For this review, take the finished solid that the model builds, in its own axes (mm). A direction names the side the tool comes from. Give positions to 0.01 mm unless a question says otherwise; leave off trailing zeros. Order: outer loops, then holes, each group sorted by start corner. A loop starts at its lowest first (then second) coordinate and runs counter-clockwise, first axis right, second up. Notation, with made-up numbers: (39, 63) - (49, 63) arc R9 cw to (49, 79) - close; hole circle Ø9 at (-17.75, 77). An arc over 180 degrees is marked (long way). Use a Markdown table: item, result. Add a question column.
1) We need section D-D on y = -27.75. Write out the cut boundary in (x, z).
2) We need section A-A on y = -23. Write out the cut boundary in (x, z), then the cut area to 3 significant figures.
3) Mouldability with a two-part tool opening along Y and no side actions: class faces 1 (the face through (1, -19.576, 7)), 2 (the face through (1.479, -15.635, 8.18)), 3 (the face through (0, -22, 9)) as released by +Y, released by -Y, zero draft, split by the parting line, or undercut.
4) Machinability: for faces 4 (the face through (1, -23, 8.769)), 5 (the face through (3, -22, 9)), which of the approach directions +Z, -Z, +X, -X, +Y, -Y give a long, thin tool a straight path to every point of the face, cutting with its end or side? Answer none if there is none.
5) We need section B-B on z = 6. Write out the cut boundary in (x, y), then the cut area to 3 significant figures.
6) We need section C-C on x = 1.3. Write out the cut boundary in (y, z).
7) Wall thickness on L1, parallel to Z at x = 1.85, y = -22.5; L2, parallel to Y at x = 2, z = 7.25; L3, parallel to Z at x = 1.3, y = -21.5: over which ranges is each line inside the solid? List them lowest first.
```python
from build123d import *

# Parameters (mm, degrees)
SKETCH1_R           = 7
SKETCH1_W           = 3
SKETCH1_H           = 6
BOSS_EXTRUDE1_DEPTH = 3


with BuildPart() as part:
    # Sketch1 → Boss-Extrude1 (new body)
    with BuildSketch(Plane(origin=(0, 0, 0), x_dir=(0, 0, -1), z_dir=(1, 0, 0))):
        with Locations((-7.268981817, -22.575682471)):
            Circle(SKETCH1_R)
        with Locations((-7.268981817, -22.575682471)):
            Rectangle(SKETCH1_W, SKETCH1_H, mode=Mode.SUBTRACT)
    extrude(amount=BOSS_EXTRUDE1_DEPTH)


solid = part.part
```
Checked values:
| question | item | result |
|---|---|---|
| 1 | outline | (0, 2.55) - (3, 2.55) - (3, 11.98) - (0, 11.98) - close |
| 2 | outline | (0, 0.28) - (3, 0.28) - (3, 5.77) - (0, 5.77) - close; (0, 8.77) - (3, 8.77) - (3, 14.26) - (0, 14.26) - close |
| 2 | area | 32.9 mm² |
| 3 | face 1 | undercut |
| 3 | face 2 | split by the parting line |
| 3 | face 3 | zero draft |
| 4 | face 4 | +X, -X |
| 4 | face 5 | +Z, -Z, +X, +Y, -Y |
| 5 | outline | (0, -29.46) - (3, -29.46) - (3, -25.58) - (0, -25.58) - close; (0, -19.58) - (3, -19.58) - (3, -15.69) - (0, -15.69) - close |
| 5 | area | 23.3 mm² |
| 6 | outline | circle Ø14 at (-22.58, 7.27); hole (-25.58, 5.77) - (-19.58, 5.77) - (-19.58, 8.77) - (-25.58, 8.77) - close |
| 7 | L1 | 0.27 to 5.77, 8.77 to 14.27 |
| 7 | L2 | -29.58 to -25.58, -19.58 to -15.58 |
| 7 | L3 | 0.35 to 5.77, 8.77 to 14.19 |
